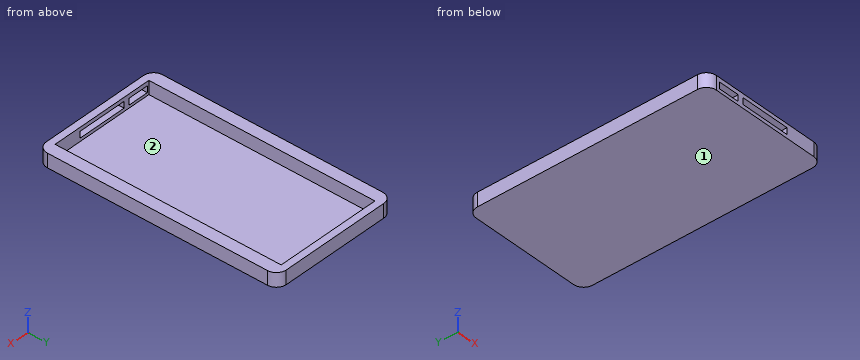
from build123d import *

# Parameters (mm, degrees)
F1_DEPTH = 0.254
F2_DEPTH = 8.509
F3_W     = 31.75
F3_H     = 4.092419
F3_W_2   = 13.322128
F4_DEPTH = 25.4


with BuildPart() as f1:
    # F0 (on Top) → F1 (new body)
    with BuildSketch(Plane.XY):
        with BuildLine():
            Line((-46.424261, 69.85), (-46.424261, 0))
            Line((-46.424261, 0), (-46.424261, -69.85))
            ThreePointArc((-46.424261, -69.85), (-44.564389, -74.340128), (-40.074261, -76.2))
            Line((-40.074261, -76.2), (30.013567, -76.2))
            ThreePointArc((30.013567, -76.2), (34.34943, -74.256845), (36.125739, -69.85))
            Line((36.125739, -69.85), (36.125739, 0))
            Line((36.125739, 0), (36.125739, 69.85))
            ThreePointArc((36.125739, 69.85), (34.34943, 74.256845), (30.013567, 76.2))
            Line((30.013567, 76.2), (-40.074261, 76.2))
            ThreePointArc((-40.074261, 76.2), (-44.564389, 74.340128), (-46.424261, 69.85))
        make_face()
        Polygon((-38.804261, 0), (-38.804261, 71.755), (28.505739, 71.755), (28.505739, 0), (28.505739, -71.755), (-38.804261, -71.755), align=None, mode=Mode.SUBTRACT)
        Polygon((28.505739, 71.755), (-38.804261, 71.755), (-38.804261, 0), (-38.804261, -71.755), (28.505739, -71.755), (28.505739, 0), align=None)
    extrude(amount=-F1_DEPTH)

    # F0 (on Top) → F2 (join)
    with BuildSketch(Plane.XY):
        with BuildLine():
            Line((-46.424261, 69.85), (-46.424261, 0))
            Line((-46.424261, 0), (-46.424261, -69.85))
            ThreePointArc((-46.424261, -69.85), (-44.564389, -74.340128), (-40.074261, -76.2))
            Line((-40.074261, -76.2), (30.013567, -76.2))
            ThreePointArc((30.013567, -76.2), (34.34943, -74.256845), (36.125739, -69.85))
            Line((36.125739, -69.85), (36.125739, 0))
            Line((36.125739, 0), (36.125739, 69.85))
            ThreePointArc((36.125739, 69.85), (34.34943, 74.256845), (30.013567, 76.2))
            Line((30.013567, 76.2), (-40.074261, 76.2))
            ThreePointArc((-40.074261, 76.2), (-44.564389, 74.340128), (-46.424261, 69.85))
        make_face()
        Polygon((-38.804261, 0), (-38.804261, 71.755), (28.505739, 71.755), (28.505739, 0), (28.505739, -71.755), (-38.804261, -71.755), align=None, mode=Mode.SUBTRACT)
    extrude(amount=F2_DEPTH)

    # F3 (on face) → F4 (cut)
    with BuildSketch(Plane.XZ.offset(76.2)):
        with Locations((-5.149261, 4.066918)):
            Rectangle(F3_W, F3_H)
        with Locations((-31.042797, 3.856391)):
            Rectangle(F3_W_2, F3_H)
    extrude(amount=-F4_DEPTH, mode=Mode.SUBTRACT)


solid = f1.part
Read the model definition and answer for the solid it produces. Units are mm, in the model's axes. Face numbers are marked on the shaded views. Round coordinates to 2 decimals unless told otherwise and drop trailing zeros. Write each loop counter-clockwise with the first axis right and the second up, starting at its lowest first coordinate (ties: lowest second). Pieces come first, ordered by that corner, then holes.
Q1. Find section B-B on x = 5.5. Determine the outline of the cut face in (y, z) (3 decimals).
Values:
outline: (-76.2, -0.254) - (76.2, -0.254) - (76.2, 8.509) - (71.755, 8.509) - (71.755, 0) - (-71.755, 0) - (-71.755, 2.021) - (-76.2, 2.021) - close; (-76.2, 6.113) - (-71.755, 6.113) - (-71.755, 8.509) - (-76.2, 8.509) - close
Q2. Straight lines are drawn through the part: line 1 (X direction, y = -36.5, z = 5); line 2 (Y direction, x = -29.5, z = 6.5) (3 decimals); line 3 (Z direction, x = 8.5, y = 39). For each, find the intervals that lie inside material, in ascending order.
Values:
line 1: x = -46.42 to -38.8, 28.51 to 36.13
line 2: y = -76.2 to -71.755, 71.755 to 76.2
line 3: z = -0.25 to 0
Q3. Find section A-A on z = 3.75. Determine the outline of the cut face in (x, y) (3 decimals).
Values:
outline: (-46.424, -69.85) arc R6.35 ccw to (-40.074, -76.2) - (-37.704, -76.2) - (-37.704, -71.755) - (-38.804, -71.755) - (-38.804, 71.755) - (28.506, 71.755) - (28.506, -71.755) - (10.726, -71.755) - (10.726, -76.2) - (30.014, -76.2) arc R6.355 ccw to (36.126, -69.85) - (36.126, 69.85) arc R6.355 ccw to (30.014, 76.2) - (-40.074, 76.2) arc R6.35 ccw to (-46.424, 69.85) - close; (-24.382, -76.2) - (-21.024, -76.2) - (-21.024, -71.755) - (-24.382, -71.755) - close
Q4. The mould has two halves that part along Y. Classify the marked faces 1 and 2: released by +Y, released by -Y, zero draft, split by the parting line, or undercut.
Values:
face 1: zero draft
face 2: undercut
Q5. Find section C-C on y = -2.5. Determine the outline of the cut face in (x, z), and give its area (3 significant figures).
Values:
outline: (-46.42, -0.25) - (36.13, -0.25) - (36.13, 8.51) - (28.51, 8.51) - (28.51, 0) - (-38.8, 0) - (-38.8, 8.51) - (-46.42, 8.51) - close
area: 151 mm2
Q6. Find section D-D on x = 24. Determine the outline of the cut face in (y, z) (3 decimals).
Values:
outline: (-76.2, -0.254) - (76.2, -0.254) - (76.2, 8.509) - (71.755, 8.509) - (71.755, 0) - (-71.755, 0) - (-71.755, 8.509) - (-76.2, 8.509) - close
Q7. Flat-ended cylindrical pins translate along their axes: P1, Ø4.5, axis at y = -73.5, z = 4, coming from the +X side; P2, Ø2, axis at y = -74.5, z = 3, coming from the -X side; P3, Ø1.2, axis at y = -73.5, z = 3, coming from the +X side. Find the tip coordinate at first contact, or state that the pin passes through.
Values:
P1: stops at x = 35.97
P2: stops at x = -45.27
P3: stops at x = 35.35
